CAD build for the part. Positions are in the model's coordinates, mm. Face numbers are marked on the shaded views. A direction names the side the tool comes from. Coordinates: 2 decimals unless noted, no trailing zeros. Loops run counter-clockwise (first coordinate to the right, second up) from the corner with the lowest first, then second, coordinate; pieces in that order, holes last. Notation, with made-up numbers: (-9, 29) -> (34, 29) arc R13 cw to (34, 53) -> close; hole circle Ø11 at (-37, 18.5). An arc over 180 degrees is marked (long way). Answer as a JSON object with one key per item and string values. Group by question number.
from build123d import *

# Parameters (mm, degrees)
SKETCH001_W      = 70
SKETCH001_H      = 10
EXTRUDE001_DEPTH = 5
SKETCH_W         = 70
SKETCH_H         = 10
SKETCH_R         = 2.1
EXTRUDE_DEPTH    = 10


with BuildPart() as extrude001:
    # Sketch001 → Extrude001 (new body)
    with BuildSketch(Plane.XY):
        with Locations((45, 0)):
            Rectangle(SKETCH001_W, SKETCH001_H)
    extrude(amount=EXTRUDE001_DEPTH)


with BuildPart() as extrude001_1:
    # Extrude001 placement: moved
    add(extrude001.part.moved(Location((0, 0, 5))))


with BuildPart() as cut:
    # Sketch → Extrude (new body)
    with BuildSketch(Plane.XY):
        with Locations((35, 0)):
            Rectangle(SKETCH_W, SKETCH_H)
        with Locations((5, 0)):
            Circle(SKETCH_R, mode=Mode.SUBTRACT)
        with BuildLine():
            ThreePointArc((15, 2.1), (12.9, 0), (15, -2.1))
            Line((15, -2.1), (65, -2.1))
            ThreePointArc((65, -2.1), (67.1, 0), (65, 2.1))
            Line((15, 2.1), (65, 2.1))
        make_face(mode=Mode.SUBTRACT)
    extrude(amount=EXTRUDE_DEPTH)

    # Cut: cut Extrude001
    add(extrude001_1.part, mode=Mode.SUBTRACT)


solid = cut.part
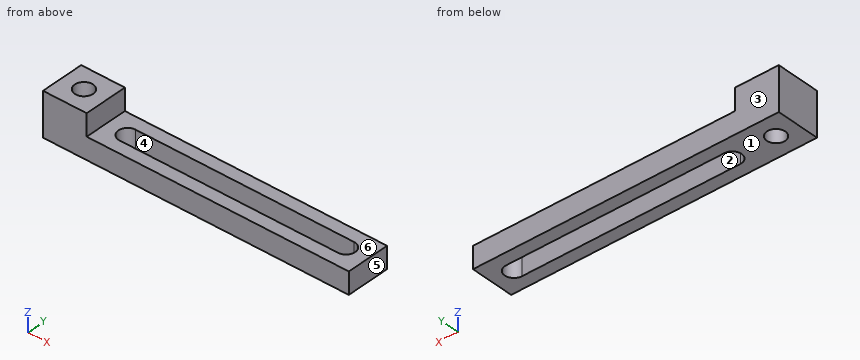
Item 1: Band-saw the part on B-B, the plane y = 0. List the corners of the cut face in (x, z).
Item 2: Band-saw the part on C-C, the plane z = 2.5. List the corners of the cut face in (x, y), and give its area (3 significant figures).
Item 3: Drill centre lines: L1, parallel to Y at x = 5, z = 6.5; L2, parallel to X at y = -0.75, z = 0.75; L3, parallel to X at y = -1.25, z = 4.5. Where is each one in solid material? Low to high.
Item 4: Band-saw the part on A-A, the plane x = 21.5. List the corners of the cut face in (y, z), and give its area (3 significant figures).
Item 5: Band-saw the part on D-D, the plane z = 8.75. List the corners of the cut face in (x, y).
Item 6: 3-axis set-ups, long thin cutter, end or side, ignore diameter. For the marked faces 5 and 6: which of +Z, -Z, +X, -X, +Y, -Y reach the whole face in a straight line?
Item 7: Flat gauge pins, fed straight in: P1, Ø6, axis at y = 1, z = 8.5, coming from the +X side; P2, Ø3, axis at x = 25, y = -4, coming from the +Z side. Where does each tip first touch, or does it go through?
Item 8: Pull direction Y, two halves, no side cores. Call the marked faces 1, 2, 3 and 4: +Y half, -Y half, draft (parallel to the pull), parting line (faces both ways), or undercut.
Reply:
{
 "1": {"outline": "(0, 0) -> (2.9, 0) -> (2.9, 10) -> (0, 10) -> close; (7.1, 0) -> (12.9, 0) -> (12.9, 5) -> (10, 5) -> (10, 10) -> (7.1, 10) -> close; (67.1, 0) -> (70, 0) -> (70, 5) -> (67.1, 5) -> close"},
 "2": {"outline": "(0, -5) -> (70, -5) -> (70, 5) -> (0, 5) -> close; hole circle Ø4.2 at (5, 0); hole (15, -2.1) -> (65, -2.1) arc R2.1 ccw to (65, 2.1) -> (15, 2.1) arc R2.1 ccw to start", "area": "462 mm²"},
 "3": {"L1": "-5 to -2.1, 2.1 to 5", "L2": "0 to 3.04, 6.96 to 13.04, 66.96 to 70", "L3": "0 to 3.31, 6.69 to 13.31, 66.69 to 70"},
 "4": {"outline": "(-5, 0) -> (-2.1, 0) -> (-2.1, 5) -> (-5, 5) -> close; (2.1, 0) -> (5, 0) -> (5, 5) -> (2.1, 5) -> close", "area": "29.0 mm²"},
 "5": {"outline": "(0, -5) -> (10, -5) -> (10, 5) -> (0, 5) -> close; hole circle Ø4.2 at (5, 0)"},
 "6": {"face 5": "+Z, -Z, +X, +Y, -Y", "face 6": "+Z, +X, +Y, -Y"},
 "7": {"P1": "x = 10", "P2": "z = 5"},
 "8": {"face 1": "draft", "face 2": "undercut", "face 3": "+Y half", "face 4": "undercut"}
}
